```python
from build123d import *

# Parameters (mm, degrees)
F0_R     = 1.15
F1_DEPTH = 3
F3_DEPTH = 3.6
F4_W     = 25
F4_H     = 5
F5_DEPTH = 1.6


with BuildPart() as f1:
    # F0 (on Top) → F1 (new body)
    with BuildSketch(Plane.XY):
        with BuildLine():
            ThreePointArc((-32.5, -29.5), (-31.767767, -31.267767), (-30, -32))
            Line((-30, -32), (30, -32))
            ThreePointArc((30, -32), (31.767767, -31.267767), (32.5, -29.5))
            Line((32.5, -29.5), (32.5, 29.5))
            ThreePointArc((32.5, 29.5), (31.767767, 31.267767), (30, 32))
            Line((30, 32), (-30, 32))
            ThreePointArc((-30, 32), (-31.767767, 31.267767), (-32.5, 29.5))
            Line((-32.5, 29.5), (-32.5, -29.5))
        make_face()
        with Locations((-30, -29.5)):
            Circle(F0_R, mode=Mode.SUBTRACT)
        with Locations((30, -29.5)):
            Circle(F0_R, mode=Mode.SUBTRACT)
        with Locations((-30, 29.5)):
            Circle(F0_R, mode=Mode.SUBTRACT)
        with Locations((30, 29.5)):
            Circle(F0_R, mode=Mode.SUBTRACT)
    extrude(amount=F1_DEPTH)

    # F2 (on face) → F3 (join)
    with BuildSketch(Plane.XY.offset(3)):
        with BuildLine():
            Line((26, 28.5), (-26, 28.5))
            ThreePointArc((-26, 28.5), (-28.828427, 27.328427), (-30, 24.5))
            Line((-30, 24.5), (-30, -24.5))
            ThreePointArc((-30, -24.5), (-28.828427, -27.328427), (-26, -28.5))
            Line((-26, -28.5), (26, -28.5))
            ThreePointArc((26, -28.5), (28.828427, -27.328427), (30, -24.5))
            Line((30, -24.5), (30, 24.5))
            ThreePointArc((30, 24.5), (28.828427, 27.328427), (26, 28.5))
        make_face()
    extrude(amount=F3_DEPTH)

    # F4 (on face) → F5 (join)
    with BuildSketch(Plane(origin=(0, 0, 0), x_dir=(1, 0, 0), z_dir=(0, 0, -1))):
        with Locations((-12.5, 34.5)):
            Rectangle(F4_W, F4_H)
        with Locations((12.5, 34.5)):
            Rectangle(F4_W, F4_H)
    extrude(amount=-F5_DEPTH)


solid = f1.part
```
For this review, take the finished solid that the model builds, in its own axes (mm). A direction names the side the tool comes from. Give positions to 0.01 mm unless a question says otherwise; leave off trailing zeros. Loops run counter-clockwise (first coordinate to the right, second up) from the corner with the lowest first, then second, coordinate; pieces in that order, holes last. Notation, with made-up numbers: M 17,22.25 L 25,22.25 A20 cw 25,43.25 Z; hole C -29.75,14 d6. An arc over 180 degrees is marked long. One line per item, written item: value. Start each with the question number.
Q1. Draft analysis for pull direction X (two halves, no side actions). For faces 1 (the face through (0, 28.5, 5)), 2 (the face through (-30, 0, 5)), 3 (the face through (30.53, 28.48, 1.48)), 4 (the face through (-29.47, 28.48, 1.48)), state which applies: released by +X, released by -X, zero draft, split by the parting line, or undercut.
Q2. Machinability: for faces 5 (the face through (-28.797, 27.359, 4.775)), 6 (the face through (0, 29, 3)), 7 (the face through (28.797, -27.359, 4.775)), 8 (the face through (28.859, 27.297, 4.775)), which of the approach directions +Z, -Z, +X, -X, +Y, -Y give a long, thin tool a straight path to every point of the face, cutting with its end or side? Answer none if there is none.
Q3. For L1, parallel to Y at x = -30, z = 0.8; L2, parallel to Y at x = -10.5, z = 5.25; L3, parallel to X at y = -17.5, z = 4.5, list the stretches that pass through material, from the lowest coordinate up.
Q4. Clearance check with flat-ended pins moving along their axes: pin 1 Ø3 at (x, y) = (30, -29.5) entering from +Z; pin 2 Ø1.8 at (y, z) = (-33.5, 1) entering from -X; pin 3 Ø1.3 at (y, z) = (-33.5, 1) entering from +X. State where each tip first meets the part, or that it passes through.
Q5. Add section A-A (y = 21). Give the boundary of the cut face in (x, z), and give its area (3 significant figures).
Q6. Add section B-B (x = -15). Give the boundary of the cut face in (y, z), and give its area (3 significant figures).
Reply:
1. face 1: zero draft
1. face 2: released by -X
1. face 3: undercut
1. face 4: undercut
2. face 5: +Z, -X, +Y
2. face 6: +Z
2. face 7: +Z, +X, -Y
2. face 8: +Z, +X, +Y
3. L1: -32 to -30.65, -28.35 to 28.35, 30.65 to 32
3. L2: -28.5 to 28.5
3. L3: -30 to 30
4. pin 1: z = 3
4. pin 2: x = -25
4. pin 3: x = 25
5. outline: M -32.5,0 L 32.5,0 L 32.5,3 L 30,3 L 30,6.6 L -30,6.6 L -30,3 L -32.5,3 Z
5. area: 411 mm²
6. outline: M -37,0 L 32,0 L 32,3 L 28.5,3 L 28.5,6.6 L -28.5,6.6 L -28.5,3 L -32,3 L -32,1.6 L -37,1.6 Z
6. area: 405 mm²
